Design review of the part built by this model. Coordinates are the model's own, in mm. Face numbers are marked on the shaded views. A direction names the side the tool comes from. Coordinates: 2 decimals unless noted, no trailing zeros. Loops run counter-clockwise (first coordinate to the right, second up) from the corner with the lowest first, then second, coordinate; pieces in that order, holes last. Notation, with made-up numbers: M 25,20.5 L 75,20.5 A22 ccw 75,52.5 Z; hole C -8.5,-24.5 d9. An arc over 180 degrees is marked long. Put each result on its own line as item: value. Start each with the question number.
(1) Clearance check with flat-ended pins moving along their axes: pin 1 (3 mm diameter, centred on x = 3, z = -2.5, fed in from +Y); pin 2 (1.4 mm diameter, centred on y = 30, z = 4.5, fed in from +X); pin 3 (1.5 mm diameter, centred on x = 5.5, y = 23, fed in from +Z); pin 4 (1.5 mm diameter, centred on x = 1, z = -1, fed in from -Y). State where each tip first meets the part, or that it passes through.
(2) Take a section at A-A, the plane x = 1.75. Give the boundary of the cut face in (y, z).
(3) The part is to be moulded in two halves that separate along X. For the marked faces 4, 5 and 6, say which applies: +X half, -X half, draft (parallel to the pull), parting line (faces both ways), or undercut.
(4) Take a section at B-B, the plane y = 7. Give the boundary of the cut face in (x, z).
(5) For the marked faces 1, 2 and 3, list the 3-axis set-ups (+Z, -Z, +X, -X, +Y, -Y) from which the entire face can be reached by the end or side of a thin tool; tool diameter is ignored.
(6) Take a section at D-D, the plane y = 15.5. Give the boundary of the cut face in (x, z), then the cut area to 3 significant figures.
(7) For probe 1 along Z at (x, y) = (0, 16); probe 2 along Z at (x, y) = (0, 5.9); probe 3 along X at (y, z) = (2.5, 0), list the stretches that pass through material, from the lowest coordinate up. Write a range as [from, to].
(8) Take a section at C-C, the plane z = -5.5. Give the boundary of the cut face in (x, y), then the cut area to 3 significant figures.
Autodesk Fusion 360 part; units mm, degrees
sketch "Sketch1" plane through (0, 0, 0) normal (0, 1, 0) x (1, 0, 0) in component "SwitchSpacer"
  arc A0 (-5.8311, -8.732) -> (-5.8573, 8.7145) centre (0, 0) cw
  arc A1 (-4.6183, -9.4298) -> (-5.8311, -8.732) centre (-5.2363, -9.1011) cw
  line L0 (-20, 3.982) -> (0, 3.982)
  arc A2 (10.4756, 0.7154) -> (10.4777, -0.6839) centre (10.5, 0.0158) cw
  arc A3 (-4.6466, 9.4159) -> (10.4756, 0.7154) centre (0, 0) cw
  arc A4 (10.4777, -0.6839) -> (-4.6183, -9.4298) centre (0, 0) cw
  arc A5 (-5.8573, 8.7145) -> (-4.6466, 9.4159) centre (-5.2637, 9.0854) cw
  line L1 (-20, -4.0237) -> (-20, 3.982)
  circle A6 centre (0, 0) radius 8
  line L2 (0, 3.982) -> (0, -4.0237)
  line L3 (0, -4.0237) -> (-20, -4.0237)
  circle A7 centre (0, 0) radius 5
  circle A8 centre (0, 0) radius 3.85
  dimension "d8" = 10
  dimension "d9" = 7.7
extrude "Extrude8" add sketch "Sketch1" along normal blind 27 contours A0 A1 L0 A2 A3 A4 A5 A6 L3 | A0 L0 A6 L3 | L0 A6 L3 A7 | L0 A6 L3 A7 | L0 L2 L3 A7 A8 | L0 L2 L3 A7 A8 in component "SwitchSpacer"
sketch "Sketch2" plane through (0, 27, 0) normal (0, 1, 0) x (-1, 0, 0) in component "SwitchSpacer"
  circle A0 centre (0, 0) radius 4
  line L0 (6.35, 6.35) -> (-6.35, 6.35)
  line L1 (-6.35, 6.35) -> (-6.35, -6.35)
  line L2 (-6.35, -6.35) -> (6.35, -6.35)
  line L3 (6.35, -6.35) -> (6.35, 6.35)
  line L4 (6.35, 6.35) -> (-6.35, -6.35) construction
  line L5 (-6.35, 6.35) -> (6.35, -6.35) construction
  line L6 (6.35, 6.35) -> (19.35, 6.35)
  line L7 (19.35, 6.35) -> (19.35, -6.35)
  line L8 (19.35, -6.35) -> (6.35, -6.35)
  line L9 (6.35, -6.35) -> (6.35, 6.35)
  circle A1 centre (0, 0) radius 6.35
  line L10 (12.5, -3.5) -> (-12.5, -3.5)
  line L11 (-12.5, -3.5) -> (-12.5, 3.5)
  line L12 (-12.5, 3.5) -> (12.5, 3.5)
  line L13 (12.5, 3.5) -> (12.5, -3.5)
  line L14 (12.5, -3.5) -> (-12.5, 3.5) construction
  line L15 (-12.5, -3.5) -> (12.5, 3.5) construction
  arc A2 (5.8573, -8.7145) -> (5.8311, 8.732) centre (0, 0) ccw
  arc A3 (5.8311, 8.732) -> (4.6183, 9.4298) centre (5.2363, 9.1011) ccw
  arc A4 (4.6183, 9.4298) -> (-10.4777, 0.6839) centre (0, 0) ccw
  arc A5 (-10.4777, 0.6839) -> (-10.4756, -0.7154) centre (-10.5, -0.0158) ccw
  arc A6 (-10.4756, -0.7154) -> (4.6466, -9.4159) centre (0, 0) ccw
  arc A7 (4.6466, -9.4159) -> (5.8573, -8.7145) centre (5.2637, -9.0854) ccw
  circle A8 centre (0, 0) radius 3.85
  dimension "d18" = 12.7
  dimension "d19" = 12.7
  dimension "d20" = 13
  dimension "d21" = 12.7
  dimension "d22" = 12.7
  dimension "d27" = 25
  dimension "d28" = 7
extrude "Extrude9" cut sketch "Sketch1" along normal blind 4 contours L0 L2 L3 A7 A8 | L0 L2 L3 A7 A8 in component "SwitchSpacer"
extrude "Extrude10" add sketch "Sketch2" along normal blind 10 contours L0 L1 L6 L12 A2 A3 A4 | L3 L6 L9 L12 A2 | L1 L2 L8 L10 A2 A6 A7 | L3 L8 L9 L10 A2 | L1 L10 L12 A4 A5 A6 in component "SwitchSpacer"
extrude "Extrude11" cut sketch "Sketch2" against normal blind 17 contours A0 L10 L12 A8 | A0 A1 L10 L12 | A0 L12 A8 | A0 A1 L12 | A0 A1 L10 | A0 L10 A8 | A0 L10 L12 A8 | A0 A1 L10 L12 | L3 L9 A1 L12 | L3 L9 A1 L10 | L3 L9 L10 L12 A2 in component "SwitchSpacer"
fillet "Fillet1" radius 3 2 edges at (-7.5989, 10, -3.5) (-7.5989, 10, 3.5) in component "SwitchSpacer"
chamfer "Chamfer1" distance 0.5 angle 45 5 edges at (-6.35, 37, -4.925) (0, 37, -6.35) (-6.35, 37, 4.925) (0, 37, 6.35) (6.35, 37, 0) in component "SwitchSpacer"
component "SwitchSpacer" placed x (1, 0, 0) y (0, 1, 0) z (0, 0, 1) at (0, 0, 0)
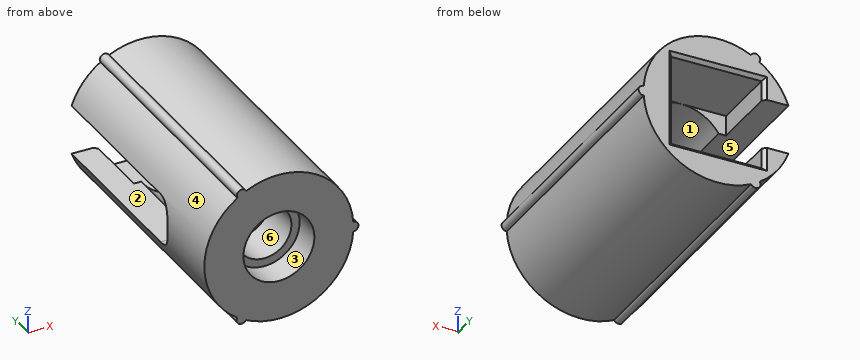
Computed values:
1. pin 1: stops at y = 10
1. pin 2: stops at x = 9.79
1. pin 3: stops at z = 9.36
1. pin 4: passes through
2. outline: M 0,-10.35 L 37,-10.35 L 37,-6.85 L 36.5,-6.35 L 27,-6.35 L 27,-6.1 L 10,-6.1 L 10,-3.43 L 4,-3.43 L 4,-4.68 L 0,-4.68 Z; M 0,4.68 L 4,4.68 L 4,3.43 L 10,3.43 L 10,6.1 L 27,6.1 L 27,6.35 L 36.5,6.35 L 37,6.85 L 37,10.35 L 0,10.35 Z
3. face 4: -X half
3. face 5: draft
3. face 6: undercut
4. outline: M -5.86,-8.71 A0.7 ccw long -4.65,-9.42 A10.5 ccw 10.48,-0.72 A0.7 ccw long 10.48,0.68 A10.5 ccw -4.62,9.43 A0.7 ccw long -5.83,8.73 A10.5 ccw Z; hole C 0,0 d7.7
5. face 1: +Y
5. face 2: -X, +Y
5. face 3: -Y
6. outline: M -9.9,-3.5 A10.5 ccw -5.86,-8.71 A0.7 ccw long -4.65,-9.42 A10.5 ccw 10.48,-0.72 A0.7 ccw long 10.48,0.68 A10.5 ccw -4.62,9.43 A0.7 ccw long -5.83,8.73 A10.5 ccw -9.9,3.5 L -5.3,3.5 A6.35 cw long -5.3,-3.5 Z
6. area: 192 mm^2
7. probe 1: z = [-10.5, -6.35], [6.35, 10.5]
7. probe 2: z = [-10.5, -3.85], [3.85, 10.5]
7. probe 3: x = [-10.5, -5], [5, 11.2]
8. outline: M -8.94,0 L 8.94,0 L 8.94,37 L 6.85,37 L 6.35,36.5 L 6.35,27 L 3.17,27 L 3.17,10 L -3.17,10 L -3.17,27 L -6.35,27 L -6.35,36.5 L -6.85,37 L -8.94,37 Z
8. area: 427 mm^2
